```python
from build123d import *

# Parameters (mm, degrees)
SKETCH1_W                         = 19
SKETCH1_H                         = 15.5
BASE_EXTRUSION_DEPTH              = 15
SKETCH2_W                         = 0.3
SKETCH2_H                         = 1.2
SKETCH2_W_2                       = 0.5
SKETCH2_H_2                       = 0.5
SKETCH2_W_3                       = 1
PINS_DEPTH                        = 4.4
SKETCH3_W                         = 0.5
SKETCH3_H                         = 1
STANDOFF_DEPTH                    = 0.5
STANDOFF_MIRROR_2_COPY_1_SKETCH_W = 0.5
STANDOFF_MIRROR_2_COPY_1_SKETCH_H = 1
STANDOFF_MIRROR_2_COPY_1_DEPTH    = 0.5
TOP_EDGE_ROUNDS_R                 = 0.75


with BuildPart() as part:
    # Sketch1 → Base Extrusion (new body)
    with BuildSketch(Plane(origin=(0, 0, 0), x_dir=(1, 0, 0), z_dir=(0, 1, 0))):
        Rectangle(SKETCH1_W, SKETCH1_H)
    extrude(amount=BASE_EXTRUSION_DEPTH)

    # Sketch2 → Pins (add)
    with BuildSketch(Plane.XZ):
        with Locations((-8.1, 0)):
            Rectangle(SKETCH2_W, SKETCH2_H)
        with Locations((-6.1, -6)):
            Rectangle(SKETCH2_W_2, SKETCH2_H_2)
        with Locations((-6.1, 6)):
            Rectangle(SKETCH2_W_2, SKETCH2_H_2)
        with Locations((6.1, 6)):
            Rectangle(SKETCH2_W_3, SKETCH2_H_2)
        with Locations((6.1, -6)):
            Rectangle(SKETCH2_W_3, SKETCH2_H_2)
    extrude(amount=PINS_DEPTH)

    # Sketch3 → Standoff (add)
    with BuildSketch(Plane.XZ):
        with Locations((-9.25, 5.75)):
            Rectangle(SKETCH3_W, SKETCH3_H)
    standoff = extrude(amount=STANDOFF_DEPTH)

    # Standoff Mirror: Standoff across plane
    add(standoff.mirror(Plane.XY))

    # Standoff Mirror 2: Standoff across plane
    add(standoff.mirror(Plane(origin=(0, 0, 0), x_dir=(0, 0, 1), z_dir=(1, 0, 0))))

    # Standoff Mirror 2 copy 1 sketch → Standoff Mirror 2 copy 1 (add)
    with BuildSketch(Plane(origin=(0, 0, 0), x_dir=(-1, 0, 0), z_dir=(0, -1, 0))):
        with Locations((-9.25, 5.75)):
            Rectangle(STANDOFF_MIRROR_2_COPY_1_SKETCH_W, STANDOFF_MIRROR_2_COPY_1_SKETCH_H)
    extrude(amount=STANDOFF_MIRROR_2_COPY_1_DEPTH)

    # Top Edge Rounds
    top_edge_rounds_edges = [part.edges().sort_by_distance(p)[0] for p in [
        (9.5, 15, 0),
        (0, 15, -7.75),
        (-9.5, 15, 0),
        (0, 15, 7.75),
    ]]
    fillet(top_edge_rounds_edges, radius=TOP_EDGE_ROUNDS_R)


solid = part.part
```
Model file for the job. Use its own axes, mm. A direction names the side the tool comes from. Coordinates: 2 decimals unless noted, no trailing zeros. Write each loop counter-clockwise with the first axis right and the second up, starting at its lowest first coordinate (ties: lowest second). Pieces come first, ordered by that corner, then holes. Notation, with made-up numbers: (53.25, 56) - (90.25, 56) arc R31 ccw to (90.25, 90) - close; hole circle Ø5 at (-1, 68.5). An arc over 180 degrees is marked (long way). One line per item, written item: value. Start each with the question number.
1. Slice it at A-A (x = 6). Write the cut outline in (y, z), plus the area to 3 significant figures.
2. Tool access for faces 1 (the flat face through (6, -2, 6.25)), 2 (the flat face through (9.5, 7, 0)), 3 (the flat face through (6, -2, -6.25)): list every direction of +Z, -Z, +X, -X, +Y, -Y with a clear straight run to the whole face (end or side of a thin tool).
3. Flat gauge pins, fed straight in: pin 1 (0.6 mm diameter, centred on x = 9.5, z = 6, fed in from -Y); pin 2 (1.3 mm diameter, centred on y = -3.5, z = 0, fed in from +X); pin 3 (8 mm diameter, centred on x = 3, z = 2.5, fed in from -Y). Where does each tip first touch, or does it go through?
4. Slice it at C-C (x = -3.5). Write the cut outline in (y, z), plus the area to 3 significant figures.
5. Probe line 1 (Y direction, x = 3.25, z = -4.5); line 2 (X direction, y = -0.75, z = -0.5). List the from-to ranges inside material, lowest first. Write a range as from..to.
6. Mould opens along X. For faces 4 (the flat face through (0, 15, 0)), 5 (the flat face through (-7.95, -2, 0)), 6 (the flat face through (-8.25, -2, 0)) say: released by +X, released by -X, zero draft, split by the parting line, or undercut.
7. Slice it at B-B (z = 4.5). Write the cut outline in (x, y), plus the area to 3 significant figures.
Answers below:
1. outline: (-4.4, -6.25) - (0, -6.25) - (0, -7.75) - (14.25, -7.75) arc R0.75 ccw to (15, -7) - (15, 7) arc R0.75 ccw to (14.25, 7.75) - (0, 7.75) - (0, 6.25) - (-4.4, 6.25) - (-4.4, 5.75) - (0, 5.75) - (0, -5.75) - (-4.4, -5.75) - close
1. area: 237 mm^2
2. face 1: +Z, +X, -X, -Y
2. face 2: +Z, -Z, +X, +Y, -Y
2. face 3: -Z, +X, -X, -Y
3. pin 1: stops at y = -0.5
3. pin 2: stops at x = -7.95
3. pin 3: stops at y = 0
4. outline: (0, -7.75) - (14.25, -7.75) arc R0.75 ccw to (15, -7) - (15, 7) arc R0.75 ccw to (14.25, 7.75) - (0, 7.75) - close
4. area: 232 mm^2
5. line 1: y = 0..15
5. line 2: x = -8.25..-7.95
6. face 4: zero draft
6. face 5: released by +X
6. face 6: released by -X
7. outline: (-9.5, 0) - (9.5, 0) - (9.5, 14.25) arc R0.75 ccw to (8.75, 15) - (-8.75, 15) arc R0.75 ccw to (-9.5, 14.25) - close
7. area: 285 mm^2
